Answer from the drawing. Dimensions are ordinates in mm from the lowest x, y and z of the part. Round coordinates to 2 decimals unless told otherwise and drop trailing zeros. Loops run counter-clockwise (first coordinate to the right, second up) from the corner with the lowest first, then second, coordinate; pieces in that order, holes last. Notation, with made-up numbers: (21, -8.75) - (59, -8.75) arc R22 ccw to (59, 0.25) - close; hole circle Ø7 at (-26.75, 14.5). An arc over 180 degrees is marked (long way). Answer as CSV lines item,"result".
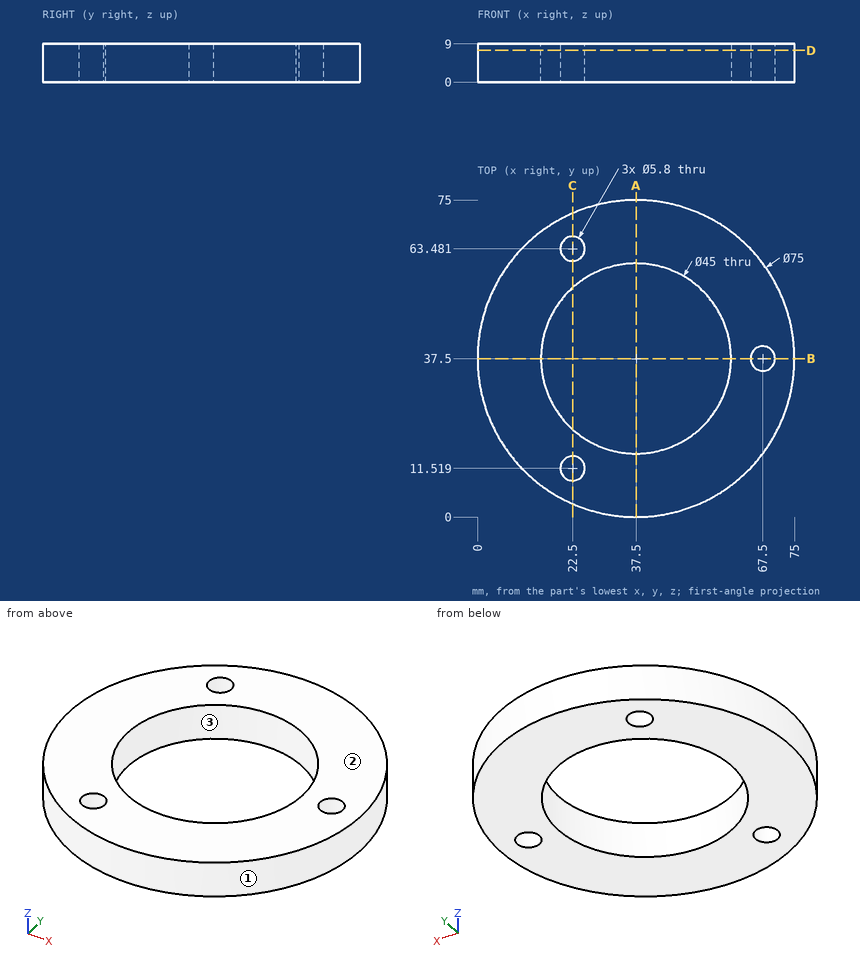
1) A cutting plane is placed at B-B, the plane y = 37.5. Determine the outline of the cut face in (x, z).
Entries:
outline,"(0, 0) - (15, 0) - (15, 9) - (0, 9) - close; (60, 0) - (64.6, 0) - (64.6, 9) - (60, 9) - close; (70.4, 0) - (75, 0) - (75, 9) - (70.4, 9) - close"
2) A cutting plane is placed at D-D, the plane z = 7.5. Determine the outline of the cut face in (x, y), plus the area to 3 significant figures.
Entries:
outline,"circle Ø75 at (37.5, 37.5); hole circle Ø45 at (37.5, 37.5); hole circle Ø5.8 at (22.5, 11.52); hole circle Ø5.8 at (22.5, 63.48); hole circle Ø5.8 at (67.5, 37.5)"
area,"2,750 mm^2"
3) Each of these flat-tipped pins is pushed along its axis until it touches: P1, Ø2, axis at x = 33, z = 6, coming from the +Y side; P2, Ø1, axis at y = 64, z = 7, coming from the -X side; P3, Ø4, axis at x = 20.5, z = 1, coming from the -Y side; P4, Ø10, axis at x = 8.5, y = 47.5, coming from the -Z side. Where does it stop, or does it pass through?
Entries:
P1,"stops at y = 74.84"
P2,"stops at x = 10.48"
P3,"stops at y = 3.13"
P4,"stops at z = 0"
4) The mould has two halves that part along Y. Classify the marked faces 1, 2 and 3: pulls with the +Y half, pulls with the -Y half, needs draft (parallel to the pull), parting line crosses it, or undercut.
Entries:
face 1,"parting line crosses it"
face 2,"needs draft"
face 3,"undercut"
5) A cutting plane is placed at A-A, the plane x = 37.5. Determine the outline of the cut face in (y, z).
Entries:
outline,"(0, 0) - (15, 0) - (15, 9) - (0, 9) - close; (60, 0) - (75, 0) - (75, 9) - (60, 9) - close"
6) A cutting plane is placed at C-C, the plane x = 22.5. Determine the outline of the cut face in (y, z).
Entries:
outline,"(3.13, 0) - (8.62, 0) - (8.62, 9) - (3.13, 9) - close; (14.42, 0) - (20.73, 0) - (20.73, 9) - (14.42, 9) - close; (54.27, 0) - (60.58, 0) - (60.58, 9) - (54.27, 9) - close; (66.38, 0) - (71.87, 0) - (71.87, 9) - (66.38, 9) - close"
7) Find the intervals of material crossed by line 1 (Y direction, x = 67.5, z = 2.5); line 2 (Y direction, x = 22.5, z = 4); line 3 (Y direction, x = 23, z = 5.25) (1 decimal), in increasing order.
Entries:
line 1,"y = 15 to 34.6, 40.4 to 60"
line 2,"y = 3.13 to 8.62, 14.42 to 20.73, 54.27 to 60.58, 66.38 to 71.87"
line 3,"y = 2.9 to 8.7, 14.4 to 20.3, 54.7 to 60.6, 66.3 to 72.1"
